Input: part model. Units: mm. Frame: model coordinates. Face numbers are marked on the shaded views. A direction names the side the tool comes from. Give positions to 0.01 mm unless a question says otherwise; leave off trailing zeros. Loops run counter-clockwise (first coordinate to the right, second up) from the corner with the lowest first, then second, coordinate; pieces in that order, holes last. Notation, with made-up numbers: (-14.5, -3) -> (16.5, -3) arc R19 ccw to (16.5, 30) -> close; hole circle Ø3 at (19, 1). An arc over 180 degrees is marked (long way). Answer as a JSON object with one key per item and string values.
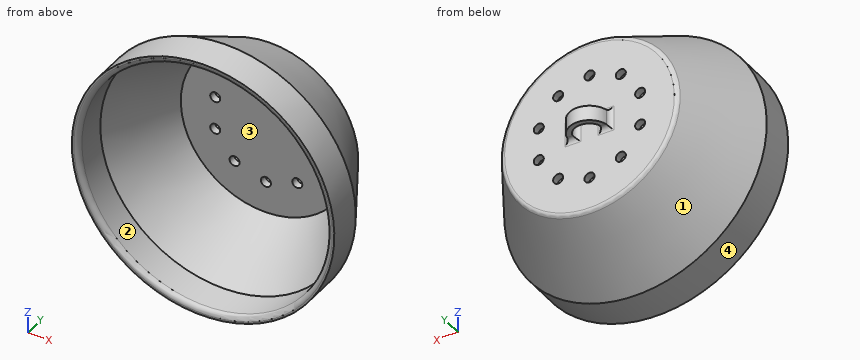
```python
from build123d import *

# Parameters (mm, degrees)
SKETCH1_R           = 26.15
SKETCH1_R_2         = 24.75
BOSS_EXTRUDE1_DEPTH = 7
SKETCH3_R           = 26.15
BOSS_EXTRUDE2_DEPTH = 15
BOSS_EXTRUDE2_TAPER = 30
SKETCH4_R           = 24.75
CUT_EXTRUDE1_DEPTH  = 13.5
CUT_EXTRUDE1_DRAFT  = -30
BOSS_EXTRUDE4_DEPTH = 1.5
FILLET2_R           = 1
CUT_EXTRUDE2_REACH  = 45.031
SKETCH6_R           = 1


with BuildPart() as part:
    # Sketch1 → Boss-Extrude1 (new body)
    with BuildSketch(Plane(origin=(0, 0, 0), x_dir=(1, 0, 0), z_dir=(0, 1, 0))):
        with Locations(Location((0, 0, 0), (0, 0, 270))):
            Circle(SKETCH1_R)
        with Locations(Location((0, 0, 0), (0, 0, 270))):
            Circle(SKETCH1_R_2, mode=Mode.SUBTRACT)
    extrude(amount=BOSS_EXTRUDE1_DEPTH)

    # Sketch3 → Boss-Extrude2 (add)
    with BuildSketch(Plane(origin=(0, 7, 0), x_dir=(1, 0, 0), z_dir=(0, 1, 0))):
        with Locations(Location((0, 0, 0), (0, 0, 270))):
            Circle(SKETCH3_R)
    extrude(amount=BOSS_EXTRUDE2_DEPTH, taper=BOSS_EXTRUDE2_TAPER)


with BuildPart() as cut_extrude1_tool:
    # Sketch4 → Cut-Extrude1 (with draft: the straight prism first)
    with BuildSketch(Plane.XZ.offset(-7)):
        with Locations(Location((0, 0, 0), (0, 0, 270))):
            Circle(SKETCH4_R)
    extrude(amount=-CUT_EXTRUDE1_DEPTH)
    # Cut-Extrude1: the draft: its side faces are tilted about the plane it starts from
    cut_extrude1_sides = [cut_extrude1_tool.faces().sort_by_distance(p)[0] for p in [
        (0, 13.75, 24.75),
    ]]
    draft(cut_extrude1_sides, Plane.XZ.offset(-7), CUT_EXTRUDE1_DRAFT)


with BuildPart() as part_1:
    add(part.part)

    # Cut-Extrude1: cut by cut_extrude1_tool
    add(cut_extrude1_tool.part, mode=Mode.SUBTRACT)

    # Sketch5 → Boss-Extrude4 (add, symmetric)
    with BuildSketch(Plane.XY):
        with BuildLine():
            Line((-4, 22), (-3, 22))
            ThreePointArc((-3, 22), (0, 25), (3, 22))
            Line((3, 22), (4, 22))
            ThreePointArc((4, 22), (0, 26), (-4, 22))
        make_face()
    extrude(amount=BOSS_EXTRUDE4_DEPTH, both=True)

    # Fillet2
    fillet2_edges = [part_1.edges().sort_by_distance(p)[0] for p in [
        (4, 22, 0),
        (-3.5, 22, -1.5),
        (-4, 22, 0),
        (-3, 22, 0),
        (3.5, 22, -1.5),
        (3, 22, 0),
        (-3.5, 22, 1.5),
        (3.5, 22, 1.5),
        (0, 0, -24.75),
        (0, 22, -17.489745962),
    ]]
    fillet(fillet2_edges, radius=FILLET2_R)

    # Sketch6 → Cut-Extrude2 (cut, up to next)
    with BuildSketch(Plane(origin=(0, 22, 0), x_dir=(1, 0, 0), z_dir=(0, 1, 0)), mode=Mode.PRIVATE) as cut_extrude2_sk1:
        with Locations(Location((0, 10.620343227, 0), (0, 0, 270))):
            Circle(SKETCH6_R)
    cut_extrude2_tool1 = extrude(cut_extrude2_sk1.sketch, amount=-CUT_EXTRUDE2_REACH, mode=Mode.PRIVATE) & part_1.part
    # Sketch6 → Cut-Extrude2 (cut, up to next)
    with BuildSketch(Plane(origin=(0, 22, 0), x_dir=(1, 0, 0), z_dir=(0, 1, 0)), mode=Mode.PRIVATE) as cut_extrude2_sk2:
        with Locations(Location((6.242481123, 8.592038157, 0), (0, 0, 270))):
            Circle(SKETCH6_R)
    cut_extrude2_tool2 = extrude(cut_extrude2_sk2.sketch, amount=-CUT_EXTRUDE2_REACH, mode=Mode.PRIVATE) & part_1.part
    # Sketch6 → Cut-Extrude2 (cut, up to next)
    with BuildSketch(Plane(origin=(0, 22, 0), x_dir=(1, 0, 0), z_dir=(0, 1, 0)), mode=Mode.PRIVATE) as cut_extrude2_sk3:
        with Locations(Location((10.100546631, 3.281866543, 0), (0, 0, 270))):
            Circle(SKETCH6_R)
    cut_extrude2_tool3 = extrude(cut_extrude2_sk3.sketch, amount=-CUT_EXTRUDE2_REACH, mode=Mode.PRIVATE) & part_1.part
    # Sketch6 → Cut-Extrude2 (cut, up to next)
    with BuildSketch(Plane(origin=(0, 22, 0), x_dir=(1, 0, 0), z_dir=(0, 1, 0)), mode=Mode.PRIVATE) as cut_extrude2_sk4:
        with Locations(Location((10.100546631, -3.281866543, 0), (0, 0, 270))):
            Circle(SKETCH6_R)
    cut_extrude2_tool4 = extrude(cut_extrude2_sk4.sketch, amount=-CUT_EXTRUDE2_REACH, mode=Mode.PRIVATE) & part_1.part
    # Sketch6 → Cut-Extrude2 (cut, up to next)
    with BuildSketch(Plane(origin=(0, 22, 0), x_dir=(1, 0, 0), z_dir=(0, 1, 0)), mode=Mode.PRIVATE) as cut_extrude2_sk5:
        with Locations(Location((6.242481123, -8.592038157, 0), (0, 0, 270))):
            Circle(SKETCH6_R)
    cut_extrude2_tool5 = extrude(cut_extrude2_sk5.sketch, amount=-CUT_EXTRUDE2_REACH, mode=Mode.PRIVATE) & part_1.part
    # Sketch6 → Cut-Extrude2 (cut, up to next)
    with BuildSketch(Plane(origin=(0, 22, 0), x_dir=(1, 0, 0), z_dir=(0, 1, 0)), mode=Mode.PRIVATE) as cut_extrude2_sk6:
        with Locations(Location((0, -10.620343227, 0), (0, 0, 270))):
            Circle(SKETCH6_R)
    cut_extrude2_tool6 = extrude(cut_extrude2_sk6.sketch, amount=-CUT_EXTRUDE2_REACH, mode=Mode.PRIVATE) & part_1.part
    # Sketch6 → Cut-Extrude2 (cut, up to next)
    with BuildSketch(Plane(origin=(0, 22, 0), x_dir=(1, 0, 0), z_dir=(0, 1, 0)), mode=Mode.PRIVATE) as cut_extrude2_sk7:
        with Locations(Location((-6.242481123, -8.592038157, 0), (0, 0, 270))):
            Circle(SKETCH6_R)
    cut_extrude2_tool7 = extrude(cut_extrude2_sk7.sketch, amount=-CUT_EXTRUDE2_REACH, mode=Mode.PRIVATE) & part_1.part
    # Sketch6 → Cut-Extrude2 (cut, up to next)
    with BuildSketch(Plane(origin=(0, 22, 0), x_dir=(1, 0, 0), z_dir=(0, 1, 0)), mode=Mode.PRIVATE) as cut_extrude2_sk8:
        with Locations(Location((-10.100546631, -3.281866543, 0), (0, 0, 270))):
            Circle(SKETCH6_R)
    cut_extrude2_tool8 = extrude(cut_extrude2_sk8.sketch, amount=-CUT_EXTRUDE2_REACH, mode=Mode.PRIVATE) & part_1.part
    # Sketch6 → Cut-Extrude2 (cut, up to next)
    with BuildSketch(Plane(origin=(0, 22, 0), x_dir=(1, 0, 0), z_dir=(0, 1, 0)), mode=Mode.PRIVATE) as cut_extrude2_sk9:
        with Locations(Location((-10.100546631, 3.281866543, 0), (0, 0, 270))):
            Circle(SKETCH6_R)
    cut_extrude2_tool9 = extrude(cut_extrude2_sk9.sketch, amount=-CUT_EXTRUDE2_REACH, mode=Mode.PRIVATE) & part_1.part
    # Sketch6 → Cut-Extrude2 (cut, up to next)
    with BuildSketch(Plane(origin=(0, 22, 0), x_dir=(1, 0, 0), z_dir=(0, 1, 0)), mode=Mode.PRIVATE) as cut_extrude2_sk10:
        with Locations(Location((-6.242481123, 8.592038157, 0), (0, 0, 270))):
            Circle(SKETCH6_R)
    cut_extrude2_tool10 = extrude(cut_extrude2_sk10.sketch, amount=-CUT_EXTRUDE2_REACH, mode=Mode.PRIVATE) & part_1.part
    add(cut_extrude2_tool1.solids().sort_by_distance((0, 22, -10.620343))[0], mode=Mode.SUBTRACT)
    add(cut_extrude2_tool2.solids().sort_by_distance((6.242481, 22, -8.592038))[0], mode=Mode.SUBTRACT)
    add(cut_extrude2_tool3.solids().sort_by_distance((10.100547, 22, -3.281867))[0], mode=Mode.SUBTRACT)
    add(cut_extrude2_tool4.solids().sort_by_distance((10.100547, 22, 3.281867))[0], mode=Mode.SUBTRACT)
    add(cut_extrude2_tool5.solids().sort_by_distance((6.242481, 22, 8.592038))[0], mode=Mode.SUBTRACT)
    add(cut_extrude2_tool6.solids().sort_by_distance((0, 22, 10.620343))[0], mode=Mode.SUBTRACT)
    add(cut_extrude2_tool7.solids().sort_by_distance((-6.242481, 22, 8.592038))[0], mode=Mode.SUBTRACT)
    add(cut_extrude2_tool8.solids().sort_by_distance((-10.100547, 22, 3.281867))[0], mode=Mode.SUBTRACT)
    add(cut_extrude2_tool9.solids().sort_by_distance((-10.100547, 22, -3.281867))[0], mode=Mode.SUBTRACT)
    add(cut_extrude2_tool10.solids().sort_by_distance((-6.242481, 22, -8.592038))[0], mode=Mode.SUBTRACT)


solid = part_1.part
```
Q1. Access query for the marked faces 1 and 2. Directions: +Z, -Z, +X, -X, +Y, -Y. A direction counts if a zero-diameter tool reaches every point of the face in a straight line with its end or side. Return the directions, or none.
Evaluation:
{"face 1": "+Y", "face 2": "-Y"}
Q2. Section C-C, the plane x = 0. Give the number of separate pieces and of enclosed holes in the cut face, then the cut area to 3 significant figures.
Evaluation:
{"separate pieces": "4", "enclosed holes": "0", "area": "108 mm2"}
Q3. Section B-B, the plane y = 4.75. Return the cut outline in (x, z).
Evaluation:
{"outline": "circle Ø52.3 at (0, 0); hole circle Ø49.5 at (0, 0)"}
Q4. Draft query along X for the marked faces 3 and 4. Return one class per face: +X half, -X half, draft (parallel to the pull), parting line (faces both ways), or undercut.
Evaluation:
{"face 3": "undercut", "face 4": "parting line"}
Q5. Ray query, line 1 along X through (y, z) = (20.75, -8); line 2 along Y through (x, z) = (-12, -10.5); line 3 along Z through (x, y) = (10, 21). Return the intervals inside material, ascending.
Evaluation:
{"line 1": "x = -16.36 to -7.05, -5.44 to 5.44, 7.05 to 16.36", "line 2": "y = 20.5 to 22", "line 3": "z = -15.05 to -4.28, -2.29 to 2.29, 4.28 to 15.05"}
Q6. Section A-A, the plane z = 0. Return the cut outline in (x, y), then the cut area to 3 significant figures.
Evaluation:
{"outline": "(-26.15, 0) -> (-25.75, 0) arc R1 ccw to (-24.75, 1) -> (-24.75, 7) -> (-16.96, 20.5) -> (16.96, 20.5) -> (24.75, 7) -> (24.75, 1) arc R1 ccw to (25.75, 0) -> (26.15, 0) -> (26.15, 7) -> (17.78, 21.5) arc R1 ccw to (16.91, 22) -> (4.9, 22) arc R1 cw to (3.92, 22.8) arc R4 ccw to (-3.92, 22.8) arc R1 cw to (-4.9, 22) -> (-16.91, 22) arc R1 ccw to (-17.78, 21.5) -> (-26.15, 7) -> close; hole (-2.6, 23.5) arc R1 ccw to (-1.73, 22) -> (1.73, 22) arc R1 ccw to (2.6, 23.5) arc R3 ccw to start", "area": "123 mm2"}
Q7. Pin query (flat end, axial travel): pin 1 (1.5 mm diameter, centred on x = -5.5, z = 2, fed in from +Y); pin 2 (4 mm diameter, centred on x = 4, y = 20, fed in from +Z); pin 3 (3 mm diameter, centred on x = -10.1, z = -3.28, fed in from -Y); pin 4 (1.6 mm diameter, centred on x = 10.1, z = -3.28, fed in from +Y). Return the tip coordinate at first contact, or that it passes through.
Evaluation:
{"pin 1": "stops at y = 22.01", "pin 2": "stops at z = 19.45", "pin 3": "stops at y = 20.5", "pin 4": "passes through"}
